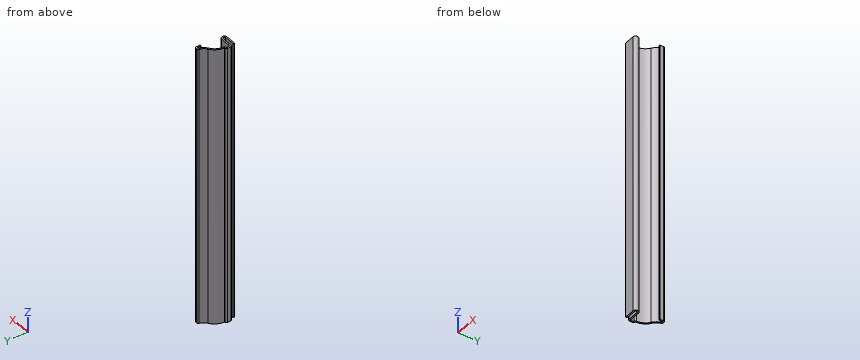
from build123d import *

# Parameters (mm, degrees)
BOSS_EXTRUDE1_DEPTH = 174.625
FILLET1_R           = 0.889


with BuildPart() as part:
    # Sketch1 → Boss-Extrude1 (new body)
    with BuildSketch(Plane.XY):
        with BuildLine():
            Line((-0.889, 15.08125), (-0.889, 17.36725))
            Line((-0.889, 17.36725), (-1.640744106, 17.36725))
            ThreePointArc((-1.640744106, 17.36725), (-2.756675468, 14.890646285), (-4.706872009, 12.99972))
            ThreePointArc((-4.706872009, 12.99972), (-7.503098361, 9.771250732), (-8.192782673, 5.55625))
            Line((-8.192782673, 5.55625), (-9.42975, 5.55625))
            Line((-9.42975, 5.55625), (-9.42975, 3.3655))
            Line((-9.42975, 3.3655), (-2.4765, 3.3655))
            ThreePointArc((-2.4765, 3.3655), (-0.79375, 1.68275), (-2.4765, 0))
            Line((-2.4765, 0), (-8.73125, 0))
            Line((-8.73125, 0), (-8.73125, 0.889))
            Line((-8.73125, 0.889), (-2.4765, 0.889))
            ThreePointArc((-2.4765, 0.889), (-1.68275, 1.68275), (-2.4765, 2.4765))
            Line((-2.4765, 2.4765), (-10.31875, 2.4765))
            Line((-10.31875, 2.4765), (-10.31875, 6.44525))
            Line((-10.31875, 6.44525), (-9.132334267, 6.44525))
            ThreePointArc((-9.132334267, 6.44525), (-8.085204479, 10.59121468), (-5.194977502, 13.742736842))
            ThreePointArc((-5.194977502, 13.742736842), (-3.292786478, 15.690706026), (-2.38125, 18.25625))
            Line((-2.38125, 18.25625), (0, 18.25625))
            Line((0, 18.25625), (0, 15.08125))
            Line((0, 15.08125), (-0.889, 15.08125))
        make_face()
    extrude(amount=-BOSS_EXTRUDE1_DEPTH)

    # Fillet1
    fillet1_edges = [part.edges().sort_by_distance(p)[0] for p in [
        (-8.192782673, 5.55625, -87.3125),
        (-10.31875, 2.4765, -87.3125),
        (-10.31875, 6.44525, -87.3125),
        (-2.38125, 18.25625, -87.3125),
        (0, 18.25625, -87.3125),
    ]]
    fillet(fillet1_edges, radius=FILLET1_R)


solid = part.part
Design review of the part built by this model. Coordinates are the model's own, in mm. Coordinates: 2 decimals unless noted, no trailing zeros. Write each loop counter-clockwise with the first axis right and the second up, starting at its lowest first coordinate (ties: lowest second). Pieces come first, ordered by that corner, then holes. Notation, with made-up numbers: (24, 61.5) -> (58, 61.5) arc R18 ccw to (58, 76.5) -> close; hole circle Ø9 at (36, 54). An arc over 180 degrees is marked (long way). Write each question's results on one line, items separated by ' | '. Start each with the question number.
(1) Take a section at A-A on x = -6.75. Write out the cut boundary in (y, z) (1 decimal).
(2) Clearance check with flat-ended pins moving along their axes: P1, Ø2, axis at y = 14.5, z = -20, coming from the -X side; P2, Ø1, axis at y = 16, z = -150, coming from the -X side; P3, Ø1.5, axis at y = 5, z = -35.5, coming from the +X side. State where each tip first meets the part, or that it passes through.
(3) Take a section at C-C on y = 8.5. Write out the cut boundary in (x, z) (3 decimals).
(4) For line 1 along Y through (x, z) = (-5.25, -126.5); line 2 along Y through (x, z) = (-6.5, -13.5); line 3 along X through (y, z) = (16.25, -161.5), list the stretches that pass through material, from the lowest coordinate up. Write a range as from..to.
(5) Take a section at B-B on z = -31. Write out the cut boundary in (x, y), and give its area (3 significant figures).
Results found:
1) outline: (0, -174.6) -> (0.9, -174.6) -> (0.9, 0) -> (0, 0) -> close; (2.5, -174.6) -> (3.4, -174.6) -> (3.4, 0) -> (2.5, 0) -> close; (11, -174.6) -> (12.4, -174.6) -> (12.4, 0) -> (11, 0) -> close
2) P1: stops at x = -5.55 | P2: stops at x = -3.42 | P3: stops at x = -8.58
3) outline: (-8.887, -174.625) -> (-7.969, -174.625) -> (-7.969, 0) -> (-8.887, 0) -> close
4) line 1: y = 0..0.89, 2.48..3.37, 12.61..13.71 | line 2: y = 0..0.89, 2.48..3.37, 11.38..12.69 | line 3: x = -2.98..-2.01, -0.89..0
5) outline: (-10.32, 3.37) arc R0.89 ccw to (-9.43, 2.48) -> (-2.48, 2.48) arc R0.79 cw to (-2.48, 0.89) -> (-8.73, 0.89) -> (-8.73, 0) -> (-2.48, 0) arc R1.68 ccw to (-2.48, 3.37) -> (-9.43, 3.37) -> (-9.43, 5.56) -> (-9.13, 5.56) arc R0.89 ccw to (-8.24, 6.45) arc R7.84 cw to (-4.71, 13) arc R7.24 ccw to (-1.64, 17.37) -> (-0.89, 17.37) -> (-0.89, 15.08) -> (0, 15.08) -> (0, 17.37) arc R0.89 ccw to (-0.89, 18.26) -> (-1.64, 18.26) arc R0.89 ccw to (-2.51, 17.57) arc R6.35 cw to (-5.19, 13.74) arc R8.73 ccw to (-9.13, 6.45) -> (-9.43, 6.45) arc R0.89 ccw to (-10.32, 5.56) -> close | area: 35.0 mm2
